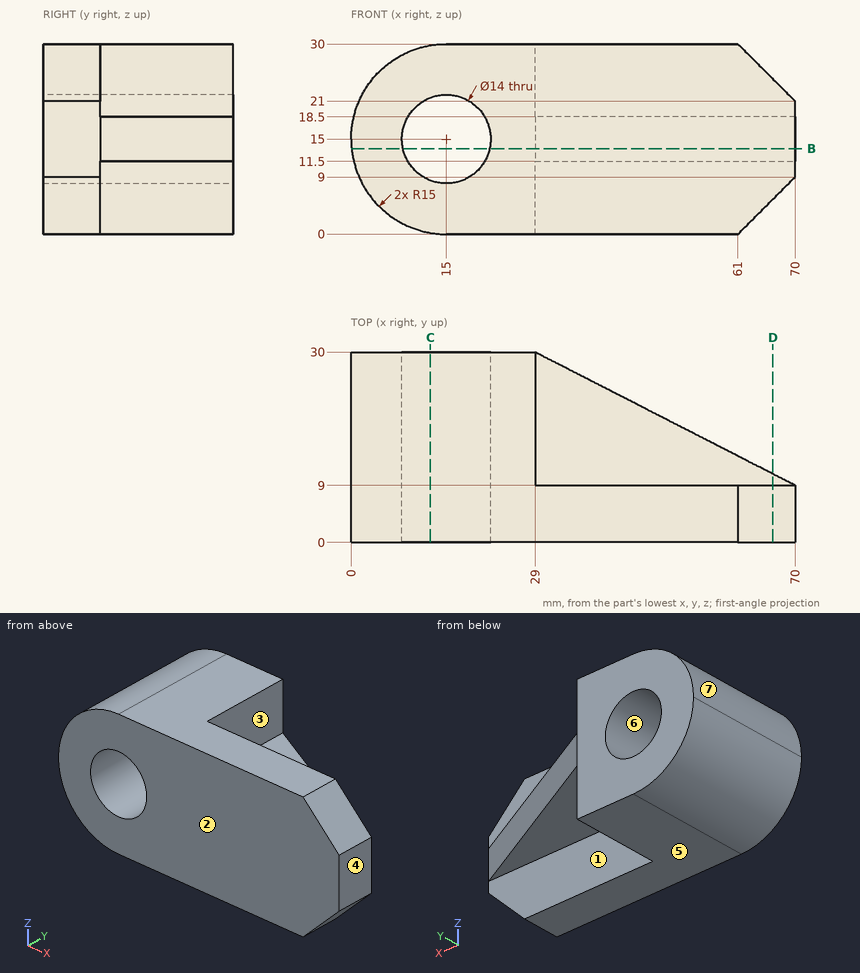
Drawing for the job (mm, zero at the part's lowest x, y, z). A direction names the side the tool comes from. Round coordinates to 2 decimals unless told otherwise and drop trailing zeros. Write each loop counter-clockwise with the first axis right and the second up, starting at its lowest first coordinate (ties: lowest second). Pieces come first, ordered by that corner, then holes. Notation, with made-up numbers: M 19.25,-7 L 43.25,-7 A10 ccw 43.25,3 Z; hole C 49.5,-13.5 d4. An arc over 180 degrees is marked long. Answer in a Markdown table with one row per item.
1. Probe L1, parallel to X at y = 7.5, z = 15; L2, parallel to Y at x = 53, z = 9.5; L3, parallel to Z at x = 35, y = 19. List the from-to ranges inside material, lowest first. Write a range as [from, to].
Geometry check:
| item | result |
|---|---|
| L1 | [0, 8], [22, 70] |
| L2 | [0, 9] |
| L3 | [11.5, 18.5] |
2. Flat gauge pins, fed straight in: P1, Ø1.5, axis at x = 32, y = 22.5, coming from the -Z side; P2, Ø6, axis at y = 21.5, z = 8, coming from the -X side; P3, Ø3, axis at x = 38.5, z = 3.5, coming from the +Y side. Where does each tip first touch, or does it go through?
Geometry check:
| item | result |
|---|---|
| P1 | z = 11.5 |
| P2 | x = 0.54 |
| P3 | y = 9 |
3. Mould opens along Z. For the marked faces 4, 5, 6 and 7 say: +Z half, -Z half, draft (parallel to the pull), parting line (faces both ways), or undercut.
Geometry check:
| item | result |
|---|---|
| face 4 | draft |
| face 5 | -Z half |
| face 6 | undercut |
| face 7 | +Z half |
4. Saw through at B-B (z = 13.5). List the corners of the cut face in (x, y) (1 decimal).
Geometry check:
| item | result |
|---|---|
| outline | M 0.1,0 L 8.2,0 L 8.2,30 L 0.1,30 Z; M 21.8,0 L 70,0 L 70,9 L 29,30 L 21.8,30 Z |
5. Saw through at C-C (x = 12.5). List the corners of the cut face in (y, z), and give its area (3 significant figures).
Geometry check:
| item | result |
|---|---|
| outline | M 0,0.21 L 30,0.21 L 30,8.46 L 0,8.46 Z; M 0,21.54 L 30,21.54 L 30,29.79 L 0,29.79 Z |
| area | 495 mm2 |
6. Saw through at D-D (x = 66.5). List the corners of the cut face in (y, z), and give its area (3 significant figures).
Geometry check:
| item | result |
|---|---|
| outline | M 0,5.5 L 9,5.5 L 9,11.5 L 10.79,11.5 L 10.79,18.5 L 9,18.5 L 9,24.5 L 0,24.5 Z |
| area | 184 mm2 |
7. Which spindle directions (+Z, -Z, +X, -X, +Y, -Y) get a long thin tool onto all of the face, cutting with end or side? Do the marked faces 1, 2 and 3. Say none if no direction does.
Geometry check:
| item | result |
|---|---|
| face 1 | -Z, +X, +Y |
| face 2 | +Z, -Z, +X, -X, -Y |
| face 3 | +Z, +X, +Y |
